Check sheet for the drawn part. Datum: minimum x, y, z corner. Units: mm. A direction names the side the tool comes from. Give positions to 0.01 mm unless a question says otherwise; leave off trailing zeros. Write each loop counter-clockwise with the first axis right and the second up, starting at its lowest first coordinate (ties: lowest second). Pieces come first, ordered by that corner, then holes. Notation, with made-up numbers: (-33, 61.5) -> (18, 61.5) arc R34 cw to (18, 96.5) -> close; hole circle Ø3 at (78, -28). An arc over 180 degrees is marked (long way). Write item = value, one per line. Start each with the question number.
1. Set-up check for the marked faces 1, 2, 3 and 4: record each of +Z, -Z, +X, -X, +Y, -Y from which the full face is reachable in a straight line by a thin tool's end or side.
2. Depth check by flat-ended pin: P1, Ø8, axis at y = 10, z = 5.5, coming from the +X side (3 decimals); P2, Ø1, axis at y = 5, z = 10.5, coming from the -X side; P3, Ø6, axis at y = 2.5, z = 26.5, coming from the -X side. Enter the tip coordinate at first touch or a pass-through.
3. Cross-section at C-C, the plane x = 28. Record the cut outline in (y, z) (3 decimals).
4. Cross-section at B-B, the plane z = 6. Record the cut outline in (x, y) (3 decimals), plus the area to 3 significant figures.
5. Thickness scan on line 1 along X through (y, z) = (8, 9.5); line 2 along Y through (x, z) = (17, 24); line 3 along X through (y, z) = (3.5, 8). Record the ranges inside material, lowest first.
6. Cross-section at A-A, the plane y = 7.62. Record the cut outline in (x, z) (3 decimals), plus the area to 3 significant figures.
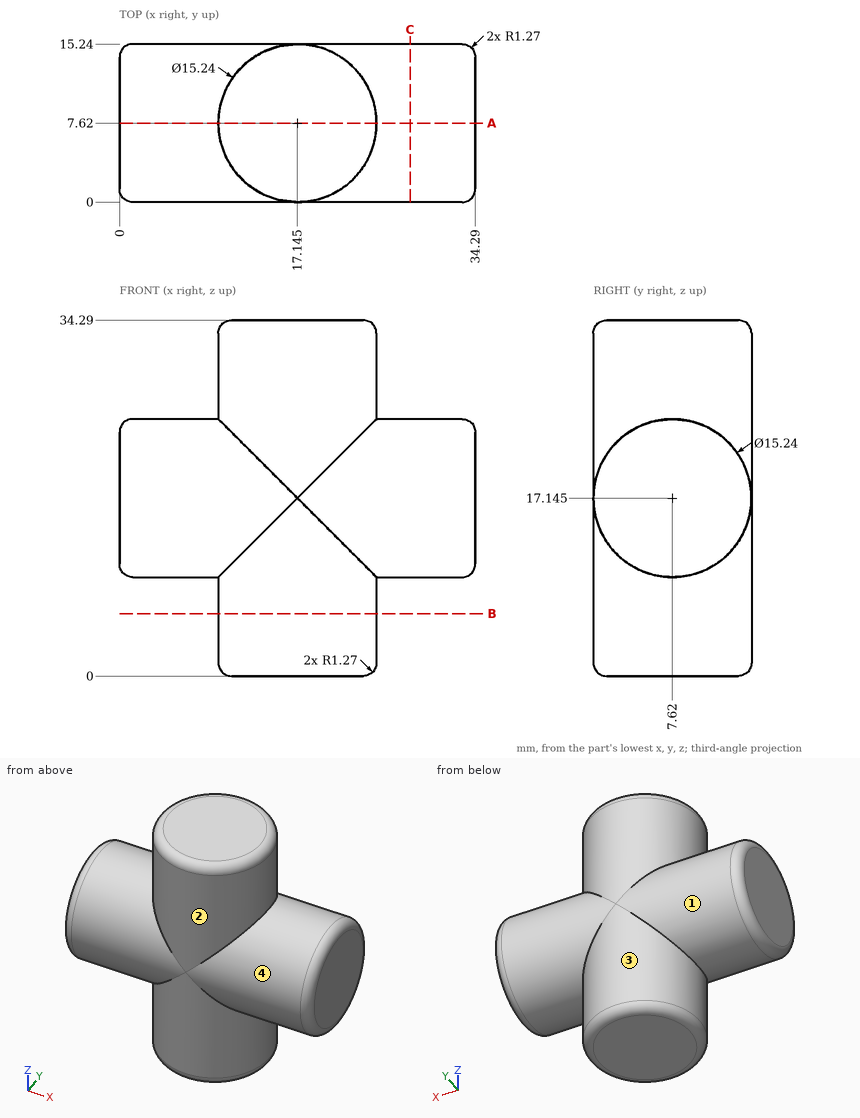
Answers:
q1.face_1 = -X
q1.face_2 = +Z
q1.face_3 = -Z
q1.face_4 = +X
q2.P1 = 24.765
q2.P2 = 0.03
q2.P3 = 9.83
q3.outline = circle Ø15.24 at (7.62, 17.145)
q4.outline = circle Ø15.24 at (17.145, 7.62)
q4.area = 182 mm^2
q5.line_1 = 9.53 to 24.76
q5.line_2 = 0 to 15.24
q5.line_3 = 10.73 to 23.56
q6.outline = (0, 10.795) arc R1.27 ccw to (1.27, 9.525) -> (9.525, 9.525) -> (9.525, 1.27) arc R1.27 ccw to (10.795, 0) -> (23.495, 0) arc R1.27 ccw to (24.765, 1.27) -> (24.765, 9.525) -> (33.02, 9.525) arc R1.27 ccw to (34.29, 10.795) -> (34.29, 23.495) arc R1.27 ccw to (33.02, 24.765) -> (24.765, 24.765) -> (24.765, 33.02) arc R1.27 ccw to (23.495, 34.29) -> (10.795, 34.29) arc R1.27 ccw to (9.525, 33.02) -> (9.525, 24.765) -> (1.27, 24.765) arc R1.27 ccw to (0, 23.495) -> close
q6.area = 810 mm^2
